Geometry check sheet. Reference: the model listing, model coordinates, mm. Coordinates: 2 decimals unless noted, no trailing zeros. Loops run counter-clockwise (first coordinate to the right, second up) from the corner with the lowest first, then second, coordinate; pieces in that order, holes last. Notation, with made-up numbers: (-35, 84) - (-8, 84) arc R23 cw to (-8, 115) - close; hole circle Ø7 at (32.5, -5). An arc over 180 degrees is marked (long way). Write each question's results on one line, items separated by ' | '. Start each with the question number.
(1) Sectioned sample at C-C (y = -28). Enter the section's corners in (x, z).
(2) Sectioned sample at B-B (z = 15). State how many separate pieces and enclosed holes the cut face has, plus the area to 3 significant figures.
(3) Go/stop test with flat-tipped pins: pin 1 Ø2 at (y, z) = (72, 20.5) entering from -X; pin 2 Ø2 at (x, z) = (31.5, 45) entering from -Y; pin 3 Ø2 at (y, z) = (71, 31.5) entering from +X; pin 4 Ø1.5 at (x, y) = (61, -72.5) entering from +Z. Record where each tip stops, or that it passes through.
(4) Sectioned sample at D-D (x = -52). Enter the section's corners in (y, z).
(5) Material ranges on probe 1 along X at (y, z) = (-43, 65.5); probe 2 along X at (y, z) = (26.5, 30.5); probe 3 along Y at (x, z) = (22, 62.5), recorded low to high.
(6) Sectioned sample at A-A (x = 0). Enter the section's corners in (y, z) (3 decimals).
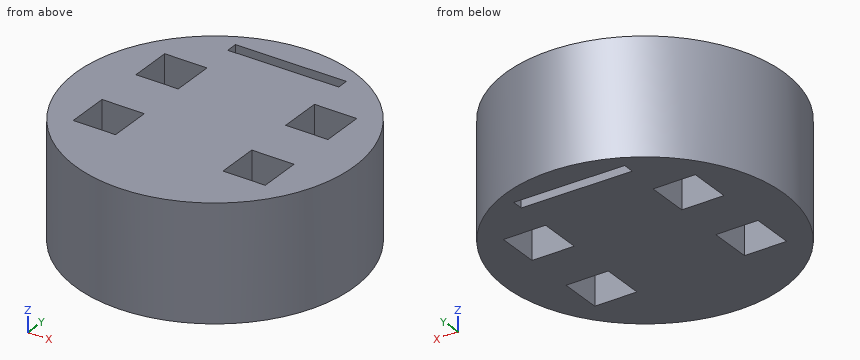
from build123d import *

# Parameters (mm, degrees)
SKETCH1_R           = 92.075
BOSS_EXTRUDE1_DEPTH = 76.2
CUT_EXTRUDE3_DEPTH  = 76.2
SKETCH8_W           = 73
SKETCH8_H           = 7.5
CUT_EXTRUDE4_DEPTH  = 76.2


with BuildPart() as part:
    # Sketch1 → Boss-Extrude1 (new body)
    with BuildSketch(Plane.XY):
        with Locations(Location((0, 0, 0), (0, 0, 180))):
            Circle(SKETCH1_R)
    extrude(amount=BOSS_EXTRUDE1_DEPTH)

    # Sketch7 → Cut-Extrude3 (cut)
    with BuildSketch(Plane(origin=(0, 0, 0), x_dir=(-1, 0, 0), z_dir=(0, 0, -1))):
        Polygon((35.148231052, 44.776310186), (35.406105201, 16.837500245), (63.344915142, 17.095374394), (63.087040993, 45.034184335), align=None)
        Polygon((63.649675499, -15.923219173), (35.710865558, -16.181093322), (35.968739707, -44.119903263), (63.907549648, -43.862029114), align=None)
        Polygon((-35.148231052, -44.776310186), (-35.406105201, -16.837500245), (-63.344915142, -17.095374394), (-63.087040993, -45.034184335), align=None)
        Polygon((-63.649675499, 15.923219173), (-35.710865558, 16.181093322), (-35.968739707, 44.119903263), (-63.907549648, 43.862029114), align=None)
    extrude(amount=-CUT_EXTRUDE3_DEPTH, mode=Mode.SUBTRACT)

    # Sketch8 → Cut-Extrude4 (cut)
    with BuildSketch(Plane.XY.offset(76.2)):
        with Locations((0, 71.06)):
            Rectangle(SKETCH8_W, SKETCH8_H)
    extrude(amount=-CUT_EXTRUDE4_DEPTH, mode=Mode.SUBTRACT)


solid = part.part
Outcome:
1) outline: (-87.71, 0) - (-63.76, 0) - (-63.76, 76.2) - (-87.71, 76.2) - close; (-35.82, 0) - (35.3, 0) - (35.3, 76.2) - (-35.82, 76.2) - close; (63.24, 0) - (87.71, 0) - (87.71, 76.2) - (63.24, 76.2) - close
2) separate pieces: 1 | enclosed holes: 5 | area: 23,000 mm2
3) pin 1: stops at x = -58.62 | pin 2: stops at y = -86.88 | pin 3: stops at x = 59.81 | pin 4: passes through
4) outline: (-75.99, 0) - (-43.97, 0) - (-43.97, 76.2) - (-75.99, 76.2) - close; (-16.03, 0) - (16.99, 0) - (16.99, 76.2) - (-16.03, 76.2) - close; (44.93, 0) - (75.99, 0) - (75.99, 76.2) - (44.93, 76.2) - close
5) probe 1: x = -81.42 to -63.9, -35.96 to 35.16, 63.11 to 81.42 | probe 2: x = -88.18 to -63.26, -35.32 to 35.81, 63.75 to 88.18 | probe 3: y = -89.41 to 67.31, 74.81 to 89.41
6) outline: (-92.075, 0) - (67.31, 0) - (67.31, 76.2) - (-92.075, 76.2) - close; (74.81, 0) - (92.075, 0) - (92.075, 76.2) - (74.81, 76.2) - close
